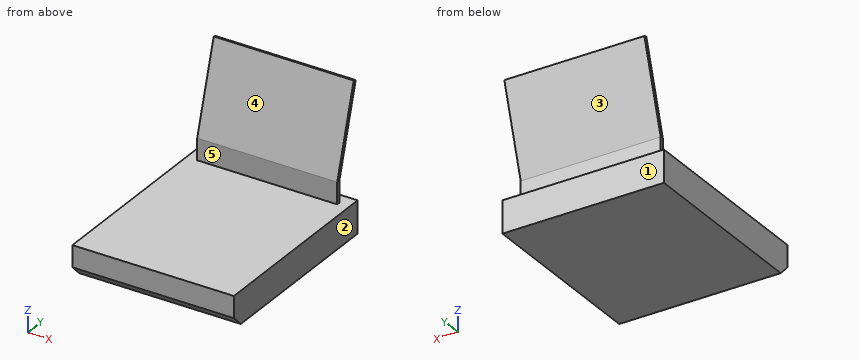
from build123d import *

# Parameters (mm, degrees)
F0_W     = 900
F0_H     = 150
F1_DEPTH = 375
F2_SIZE  = 50
F4_DEPTH = 325


with BuildPart() as f1:
    # F0 (on Right) → F1 (new body, symmetric)
    with BuildSketch(Plane.YZ):
        Rectangle(F0_W, F0_H)
    extrude(amount=F1_DEPTH, both=True)

    # F2
    f2_edges = [f1.edges().sort_by_distance(p)[0] for p in [
        (0, -450, -75),
    ]]
    chamfer(f2_edges, length=F2_SIZE)

    # F3 (on Right) → F4 (join, symmetric)
    with BuildSketch(Plane.YZ):
        Polygon((380, 175), (380, 75), (395, 75), (395, 172.798467), (514.191467, 570.103357), (500, 575), align=None)
    extrude(amount=F4_DEPTH, both=True)


solid = f1.part
Verification items for the finished model (mm, model axes). Face numbers are marked on the shaded views. A direction names the side the tool comes from. Give positions to 0.01 mm unless a question says otherwise; leave off trailing zeros. Write each loop counter-clockwise with the first axis right and the second up, starting at its lowest first coordinate (ties: lowest second). Pieces come first, ordered by that corner, then holes. Notation, with made-up numbers: M 28,-29 L 56,-29 A21 cw 56,6 Z; hole C 42.5,42.5 d10. An arc over 180 degrees is marked long. Put each result on its own line as item: value. Start each with the question number.
1. Section check B-B (y = -42.5). Record the cut outline in (x, z).
2. Section check A-A (x = -141). Record the cut outline in (y, z).
3. Section check C-C (z = 230). Record the cut outline in (x, y), and give its area (3 significant figures).
4. Draft check along Z on the marked faces 3, 4 and 5. Enter one of: +Z half, -Z half, draft (parallel to the pull), parting line (faces both ways), or undercut.
5. Scan lines: line 1 along Y through (x, z) = (264.5, 148.5); line 2 along Z through (x, y) = (-333, -242); line 3 along Y through (x, z) = (68.5, 299). Record each from-to range of solid material in increasing order. Write a range as [from, to].
6. Go/stop test with flat-tipped pins: pin 1 Ø10 at (x, z) = (130.5, 126.5) entering from -Y; pin 2 Ø3 at (x, z) = (-284.5, 349.5) entering from +Y; pin 3 Ø2 at (x, z) = (170, 117.5) entering from +Y. Record where each tip stops, or that it passes through.
7. Set-up check for the marked faces 1 and 2: record each of +Z, -Z, +X, -X, +Y, -Y from which the full face is reachable in a straight line by a thin tool's end or side.
Answer list:
1. outline: M -375,-75 L 375,-75 L 375,75 L -375,75 Z
2. outline: M -450,-25 L -400,-75 L 450,-75 L 450,75 L 395,75 L 395,172.8 L 514.19,570.1 L 500,575 L 380,175 L 380,75 L -450,75 Z
3. outline: M -325,396.5 L 325,396.5 L 325,412.16 L -325,412.16 Z
3. area: 10,200 mm2
4. face 3: undercut
4. face 4: +Z half
4. face 5: draft
5. line 1: [380, 395]
5. line 2: [-75, 75]
5. line 3: [417.2, 432.86]
6. pin 1: y = 380
6. pin 2: y = 448.46
6. pin 3: y = 395
7. face 1: -Z, +X, -X, +Y
7. face 2: +Z, -Z, +X, +Y, -Y
